Autodesk Inventor part; units mm, degrees
ref_plane "YZ Plane" through (0, 0, 0) normal (1, 0, 0) x (0, 1, 0)
ref_plane "XZ Plane" through (0, 0, 0) normal (0, 1, 0) x (-1, 0, 0)
ref_plane "XY Plane" through (0, 0, 0) normal (0, 0, 1) x (1, 0, 0)
sketch "Sketch1" plane through (0, 0, 0) normal (0, 0, 1) x (1, 0, 0)
  line L0 (-4.2367, 4.9428) -> (8.4633, 4.9428)
  line L1 (8.4633, 4.9428) -> (8.4633, -7.7572)
  line L2 (8.4633, -7.7572) -> (-4.2367, -7.7572)
  line L3 (-4.2367, -7.7572) -> (-4.2367, 4.9428)
  point P0 (0, 0)
  dimension "d0" = 12.7
  dimension "d1" = 12.7
extrude "Extrusion1" add sketch "Sketch1" along normal blind 6.35
sketch "Sketch2" plane through (0, 0, 6.35) normal (0, 0, 1) x (1, 0, 0)
  line L0 (-4.2367, -7.7572) -> (8.4633, -7.7572)
  line L1 (0.5135, -7.7572) -> (4.1203, -7.7572)
  line L2 (4.1203, -7.7572) -> (4.1203, 4.9428)
  line L3 (8.4633, 4.9428) -> (-4.2367, 4.9428)
  line L4 (4.1203, 4.9428) -> (0.5135, 4.9428)
  line L5 (0.5135, -7.7572) -> (0.5135, 4.9428)
  line L6 (0.5135, 4.9428) -> (-4.2367, 4.9428)
  line L7 (-4.2367, 4.9428) -> (-4.2367, -7.7572)
  line L8 (-4.2367, -7.7572) -> (0.5135, -7.7572)
  line L9 (0.5135, -7.7572) -> (0.5135, 4.9428)
  line L10 (4.1203, 4.9428) -> (8.4633, 4.9428)
  line L11 (8.4633, 4.9428) -> (8.4633, -7.7572)
  line L12 (8.4633, -7.7572) -> (4.1203, -7.7572)
  line L13 (4.1203, -7.7572) -> (4.1203, 4.9428)
  point P0 (0, 0)
  dimension "d4" = 3.6068
extrude "Extrusion2" add sketch "Sketch2" along normal blind 3.6068 contours L7 L3 L5 L0 | L2 L3 L11 L0
sketch "Sketch3" plane through (0, 0, 6.35) normal (0, 0, 1) x (1, 0, 0)
  line L0 (4.1203, 4.9428) -> (0.5135, 4.9428)
  line L1 (4.1203, 4.9428) -> (4.1203, -7.7572)
  line L2 (0.5135, 4.9428) -> (4.1203, 4.9428)
  line L3 (4.1203, 4.9428) -> (4.1203, 3.9157)
  line L4 (4.1203, 3.9157) -> (0.5135, 3.9157)
  line L5 (0.5135, 3.9157) -> (0.5135, 4.9428)
  point P0 (0, 0)
extrude "Extrusion3" add sketch "Sketch3" along normal blind 3.6068
sketch "Sketch4" plane through (0, 0, 9.9568) normal (0, 0, 1) x (1, 0, 0)
  line L0 (0.5135, -7.7572) -> (0.5135, 3.9157)
  line L1 (0.5135, 3.9157) -> (11.3187, 3.9157) construction
  line L2 (4.1203, -7.7572) -> (4.1203, 3.9157)
  line L3 (-4.2367, 4.9428) -> (-4.2367, -7.7572)
  line L4 (8.4633, 4.9428) -> (-4.2367, 4.9428)
  line L5 (8.4633, -7.7572) -> (8.4633, 4.9428)
  line L6 (8.4633, -6.0235) -> (8.4633, -1.9417)
  line L7 (-4.2367, -2.4282) -> (-4.2367, -6.55)
  line L8 (8.4633, -4.1258) -> (8.4633, -3.8394)
  line L9 (-4.2367, -4.6399) -> (-4.2367, -4.3516)
  line L10 (0.5135, 3.9157) -> (8.4633, -4.0341) construction
  line L11 (0.5135, 3.9157) -> (11.7563, 3.9157) construction
  line L12 (4.1203, 3.9157) -> (-3.8295, -4.0341) construction
  line L13 (4.1203, 3.9157) -> (15.3631, 3.9157) construction
  line L14 (4.1203, 3.9157) -> (5.1474, 4.9428) construction
  line L15 (0.5135, 3.9157) -> (-0.5135, 4.9428) construction
  line L16 (-0.5854, 4.8709) -> (8.4633, -4.1778)
  line L17 (8.4633, -3.8904) -> (0.0898, 4.4832)
  line L18 (0.0898, 4.4832) -> (-0.3699, 4.9428)
  line L19 (-0.5854, 4.8709) -> (-0.6572, 4.9428)
  line L20 (-3.6868, -4.0351) -> (5.3778, 5.0295)
  line L21 (4.5252, 4.4643) -> (-4.2367, -4.2976)
  line L22 (-3.6868, -4.0351) -> (-4.2367, -4.585)
  line L23 (-4.2367, -4.2976) -> (-4.2367, -4.585)
  line L24 (5.3778, 5.0295) -> (5.0904, 5.0295)
  line L25 (5.0904, 5.0295) -> (4.5252, 4.4643)
  point P0 (0, 0)
  dimension "d22" = 45
  dimension "d23" = 135
  dimension "d24" = 0.2032
  dimension "d25" = 0.2032
extrude "Extrusion7" cut sketch "Sketch4" against normal blind 5.08 contours L20 L22 L3 L21 L0 | L0 L21 L16 L20 | L20 L17 L2 L16 | L16 L21 L17 L20 | L16 L19 L4 L18 L17 L21 | L2 L17 L5 L16 | L17 L21 L25 L4 L20 | L4 L25 L24 L20
sketch "Sketch7" plane through (0, 0, 9.9568) normal (0, 0, 1) x (1, 0, 0)
  point P0 (0, 0)
properties part number "crosspiecejig"
Check sheet for the modelled part. Datum: model origin and axes. Units: mm. A direction names the side the tool comes from. Give positions to 0.01 mm unless a question says otherwise; leave off trailing zeros. Order: outer loops, then holes, each group sorted by start corner. A loop starts at its lowest first (then second) coordinate and runs counter-clockwise, first axis right, second up. Notation, with made-up numbers: (74, 70.25) - (124, 70.25) arc R25 cw to (124, 88.25) - close; hole circle Ø6 at (7, 14). An arc over 180 degrees is marked (long way). Answer as CSV lines item,"result".
1. Section check D-D (y = 3). Record the boundary of the cut face in (x, z).
Result sheet:
outline,"(-4.24, 0) - (8.46, 0) - (8.46, 9.96) - (4.12, 9.96) - (4.12, 6.35) - (3.35, 6.35) - (3.35, 4.88) - (3.06, 4.88) - (3.06, 6.35) - (1.57, 6.35) - (1.57, 4.88) - (1.29, 4.88) - (1.29, 6.35) - (0.51, 6.35) - (0.51, 9.96) - (-4.24, 9.96) - close"
2. Section check A-A (z = 7.5). State how many separate pieces and enclosed holes the cut face has, then the cut area to 3 significant figures.
Result sheet:
separate pieces,"5"
enclosed holes,"0"
area,"116 mm²"
3. Tool access check on faces 1 (the face through (4.12, 2, 8)), 2 (the face through (4.28, 4.22, 6.89)), 3 (the face through (-2, 1, 9.957)). Record the directions out of +Z, -Z, +X, -X, +Y, -Y that give a thin tool (end or side, any length) a straight path to the whole face; none if there is none.
Result sheet:
face 1,"+Z, -Y"
face 2,"+Z"
face 3,"+Z, +X, -X, +Y, -Y"
4. Mould release check, pull along X, two halves, no side actions. Record for faces 4 (the face through (6.03, -1.745, 7.452)), 5 (the face through (2, -1, 0)): released by +X, released by -X, zero draft, split by the parting line, or undercut.
Result sheet:
face 4,"undercut"
face 5,"zero draft"
5. Section check B-B (y = -6.75). Record the boundary of the cut face in (x, z).
Result sheet:
outline,"(-4.24, 0) - (8.46, 0) - (8.46, 9.96) - (4.12, 9.96) - (4.12, 6.35) - (0.51, 6.35) - (0.51, 9.96) - (-4.24, 9.96) - close"
6. Go/stop test with flat-tipped pins: P1, Ø0.8, axis at x = 3, y = 2, coming from the +Z side; P2, Ø4, axis at x = 2.5, y = -3, coming from the +Z side; P3, Ø1, axis at x = 2, z = 8.5, coming from the -Y side. Record where each tip stops, or that it passes through.
Result sheet:
P1,"z = 6.35"
P2,"z = 9.96"
P3,"y = 3.92"
7. Scan lines: probe 1 along X at (y, z) = (-1.5, 5.25); probe 2 along X at (y, z) = (2, 8.5); probe 3 along X at (y, z) = (-2.5, 8). Record each from-to range of solid material in increasing order. Write a range as from..to.
Result sheet:
probe 1,"-4.24..-1.44, -1.15..5.79, 6.07..8.46"
probe 2,"-4.24..0.51, 4.12..8.46"
probe 3,"-4.24..-2.44, -2.15..0.51, 4.12..6.79, 7.07..8.46"
8. Section check C-C (x = 3.5). Record the boundary of the cut face in (y, z), then the cut area to 3 significant figures.
Result sheet:
outline,"(-7.76, 0) - (4.94, 0) - (4.94, 9.96) - (3.92, 9.96) - (3.92, 6.35) - (3.44, 6.35) - (3.44, 4.88) - (3.15, 4.88) - (3.15, 6.35) - (1.07, 6.35) - (1.07, 4.88) - (0.79, 4.88) - (0.79, 6.35) - (-7.76, 6.35) - close"
area,"83.5 mm²"
